from build123d import *

# Parameters (mm, degrees)
SKETCH2_W           = 50.8
SKETCH2_H           = 50.8
SKETCH2_W_2         = 44.45
SKETCH2_H_2         = 44.45
BOSS_EXTRUDE1_DEPTH = 127
SKETCH4_W           = 44.45
SKETCH4_H           = 63.5
CUT_EXTRUDE1_DEPTH  = 23.368
SKETCH5_R           = 3.175
SKETCH5_W           = 42.418
SKETCH5_H           = 42.418
CUT_EXTRUDE2_DEPTH  = 100.130759523


with BuildPart() as part:
    # Sketch2 → Boss-Extrude1 (new body)
    with BuildSketch(Plane.XY):
        Rectangle(SKETCH2_W, SKETCH2_H)
        Rectangle(SKETCH2_W_2, SKETCH2_H_2, mode=Mode.SUBTRACT)
    extrude(amount=BOSS_EXTRUDE1_DEPTH)

    # Sketch4 → Cut-Extrude1 (cut)
    with BuildSketch(Plane(origin=(0, 25.4, 0), x_dir=(1, 0, 0), z_dir=(0, 1, 0))):
        with Locations((0, -31.75)):
            Rectangle(SKETCH4_W, SKETCH4_H)
    extrude(amount=-CUT_EXTRUDE1_DEPTH, mode=Mode.SUBTRACT)

    # Sketch5 → Cut-Extrude2 (cut)
    with BuildSketch(Plane.ZY.offset(25.4)):
        with Locations(Location((20.828, 0, 0), (0, 0, 270))):
            Circle(SKETCH5_R)
        with Locations((72.009, 0)):
            Rectangle(SKETCH5_W, SKETCH5_H)
    extrude(amount=-CUT_EXTRUDE2_DEPTH, mode=Mode.SUBTRACT)


solid = part.part
Model file for the job. Use its own axes, mm. A direction names the side the tool comes from. Give positions to 0.01 mm unless a question says otherwise; leave off trailing zeros. Loops run counter-clockwise (first coordinate to the right, second up) from the corner with the lowest first, then second, coordinate; pieces in that order, holes last.
1) Wall check: line 1 (Z direction, x = -23.1, y = 0); line 2 (Y direction, x = 18, z = 117) (3 decimals). Give the ranges that are in metal, low to high.
2) Saw through at A-A (x = 2). Write the cut outline in (y, z) (3 decimals).
3) Tool access for faces 5 (the flat face through (-23, 0, 127)), 6 (the flat face through (0, 24, 63.5)), 7 (the flat face through (24, 0, 50.8)): list every direction of +Z, -Z, +X, -X, +Y, -Y with a clear straight run to the whole face (end or side of a thin tool).
4) Flat gauge pins, fed straight in: pin 1 Ø5 at (x, z) = (-16.5, 55) entering from +Y (3 decimals); pin 2 Ø3 at (x, y) = (6, -19.5) entering from -Z (1 decimal); pin 3 Ø1 at (x, y) = (9.5, 24.5) entering from -Z. Where does each tip first touch, or does it go through?
5) Saw through at B-B (z = 78). Write the cut outline in (x, y) (3 decimals), plus the area to 3 significant figures.
6) Saw through at D-D (y = -9). Write the cut outline in (x, z) (3 decimals), plus the area to 3 significant figures.
7) Pull direction X, two halves, no side cores. Call faces 1 (the flat face through (0, 22.225, 95)), 2 (the flat face through (0, -22.225, 63)), 3 (the flat face through (-25.4, 0, 48)), 4 (the flat face through (-24, 0, 50.8)): +X half, -X half, draft (parallel to the pull), parting line (faces both ways), or undercut.
8) Saw through at C-C (y = 0). Write the cut outline in (x, z) (3 decimals).
Answer block:
1. line 1: z = 0 to 17.65, 24 to 50.8, 93.22 to 127
1. line 2: y = -25.4 to -22.225, 22.225 to 25.4
2. outline: (-25.4, 0) - (-22.225, 0) - (-22.225, 127) - (-25.4, 127) - close; (22.225, 63.5) - (25.4, 63.5) - (25.4, 127) - (22.225, 127) - close
3. face 5: +Z, +X, -X, +Y, -Y
3. face 6: -Z, +Y
3. face 7: +X, -X
4. pin 1: stops at y = -22.225
4. pin 2: passes through
4. pin 3: stops at z = 63.5
5. outline: (-25.4, -25.4) - (25.4, -25.4) - (25.4, -21.209) - (22.225, -21.209) - (22.225, -22.225) - (-22.225, -22.225) - (-22.225, -21.209) - (-25.4, -21.209) - close; (-25.4, 21.209) - (-22.225, 21.209) - (-22.225, 22.225) - (22.225, 22.225) - (22.225, 21.209) - (25.4, 21.209) - (25.4, 25.4) - (-25.4, 25.4) - close
5. area: 335 mm2
6. outline: (-25.4, 0) - (-22.225, 0) - (-22.225, 50.8) - (-25.4, 50.8) - close; (-25.4, 93.218) - (-22.225, 93.218) - (-22.225, 127) - (-25.4, 127) - close; (22.225, 0) - (25.4, 0) - (25.4, 50.8) - (22.225, 50.8) - close; (22.225, 93.218) - (25.4, 93.218) - (25.4, 127) - (22.225, 127) - close
6. area: 537 mm2
7. face 1: undercut
7. face 2: undercut
7. face 3: -X half
7. face 4: draft
8. outline: (-25.4, 0) - (-22.225, 0) - (-22.225, 17.653) - (-25.4, 17.653) - close; (-25.4, 24.003) - (-22.225, 24.003) - (-22.225, 50.8) - (-25.4, 50.8) - close; (-25.4, 93.218) - (-22.225, 93.218) - (-22.225, 127) - (-25.4, 127) - close; (22.225, 0) - (25.4, 0) - (25.4, 17.653) - (22.225, 17.653) - close; (22.225, 24.003) - (25.4, 24.003) - (25.4, 50.8) - (22.225, 50.8) - close; (22.225, 93.218) - (25.4, 93.218) - (25.4, 127) - (22.225, 127) - close
